Design review of the part built by this model. Coordinates are the model's own, in mm. Face numbers are marked on the shaded views. Give positions to 0.01 mm unless a question says otherwise; leave off trailing zeros. Write each loop counter-clockwise with the first axis right and the second up, starting at its lowest first coordinate (ties: lowest second). Pieces come first, ordered by that corner, then holes. Notation, with made-up numbers: (88, 13.5) -> (147, 13.5) arc R17 ccw to (147, 34.5) -> close; hole circle Ø7 at (29.5, 23.25). An arc over 180 degrees is marked (long way). Use CSV: the item, a comma, the result in double quotes.
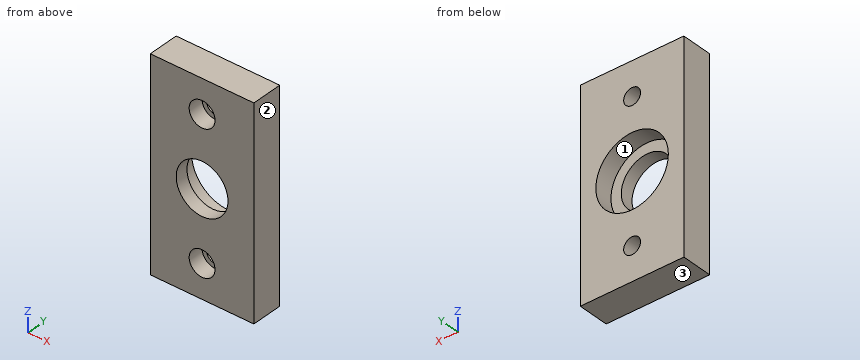
```python
from build123d import *

# Parameters (mm, degrees)
F0_W     = 40
F0_H     = 80
F0_R     = 3.25
F0_R_2   = 10
F1_DEPTH = 12
F2_R     = 5
F3_DEPTH = 6
F4_R     = 14
F5_DEPTH = 7


with BuildPart() as f1:
    # F0 (on Front) → F1 (new body)
    with BuildSketch(Plane.XZ):
        with Locations((20, 40)):
            Rectangle(F0_W, F0_H)
        with Locations((20, 13)):
            Circle(F0_R, mode=Mode.SUBTRACT)
        with Locations((20, 40)):
            Circle(F0_R_2, mode=Mode.SUBTRACT)
        with Locations((20, 67)):
            Circle(F0_R, mode=Mode.SUBTRACT)
    extrude(amount=F1_DEPTH)

    # F2 (on face) → F3 (cut)
    with BuildSketch(Plane.XZ.offset(12)):
        with Locations((20, 67)):
            Circle(F2_R)
        with Locations((20, 13)):
            Circle(F2_R)
    extrude(amount=-F3_DEPTH, mode=Mode.SUBTRACT)

    # F4 (on face) → F5 (cut)
    with BuildSketch(Plane(origin=(0, 0, 0), x_dir=(-1, 0, 0), z_dir=(0, 1, 0))):
        with Locations((-20, 40)):
            Circle(F4_R)
    extrude(amount=-F5_DEPTH, mode=Mode.SUBTRACT)


solid = f1.part
```
(1) Take a section at A-A (z = 40). Write out the cut boundary in (x, y), then the cut area to 3 significant figures.
Established:
outline,"(0, -12) -> (10, -12) -> (10, -7) -> (6, -7) -> (6, 0) -> (0, 0) -> close; (30, -12) -> (40, -12) -> (40, 0) -> (34, 0) -> (34, -7) -> (30, -7) -> close"
area,"184 mm2"
(2) Take a section at B-B (y = -2). Write out the cut boundary in (x, z), then the cut area to 3 significant figures.
Established:
outline,"(0, 0) -> (40, 0) -> (40, 80) -> (0, 80) -> close; hole circle Ø28 at (20, 40); hole circle Ø6.5 at (20, 13); hole circle Ø6.5 at (20, 67)"
area,"2,520 mm2"
(3) Mouldability with a two-part tool opening along Z and no side actions: class the marked faces 1, 2 and 3 as +Z half, -Z half, draft (parallel to the pull), parting line (faces both ways), or undercut.
Established:
face 1,"undercut"
face 2,"draft"
face 3,"-Z half"
(4) Clearance check with flat-ended pins moving along their axes: pin 1 (12 mm diameter, centred on x = 20, z = 40, fed in from -Y); pin 2 (8.5 mm diameter, centred on x = 17, z = 34, fed in from +Y). State where each tip first meets the part, or that it passes through.
Established:
pin 1,"passes through"
pin 2,"stops at y = -7"
(5) Take a section at C-C (x = 20). Write out the cut boundary in (y, z), then the cut area to 3 significant figures.
Established:
outline,"(-12, 0) -> (0, 0) -> (0, 9.75) -> (-6, 9.75) -> (-6, 8) -> (-12, 8) -> close; (-12, 18) -> (-6, 18) -> (-6, 16.25) -> (0, 16.25) -> (0, 26) -> (-7, 26) -> (-7, 30) -> (-12, 30) -> close; (-12, 50) -> (-7, 50) -> (-7, 54) -> (0, 54) -> (0, 63.75) -> (-6, 63.75) -> (-6, 62) -> (-12, 62) -> close; (-12, 72) -> (-6, 72) -> (-6, 70.25) -> (0, 70.25) -> (0, 80) -> (-12, 80) -> close"
area,"466 mm2"
(6) Take a section at D-D (z = 17). Write out the cut boundary in (x, y).
Established:
outline,"(0, -12) -> (17, -12) -> (17, -6) -> (23, -6) -> (23, -12) -> (40, -12) -> (40, 0) -> (0, 0) -> close"
(7) For line 1 along Z through (x, y) = (20, -2.25); line 2 along Z through (x, y) = (20, -9.8); line 3 along X through (y, z) = (-3, 67), list the stretches that pass through material, from the lowest coordinate up. Write a range as [from, to].
Established:
line 1,"z = [0, 9.75], [16.25, 26], [54, 63.75], [70.25, 80]"
line 2,"z = [0, 8], [18, 30], [50, 62], [72, 80]"
line 3,"x = [0, 16.75], [23.25, 40]"
